CAD build for the part. Positions are in the model's coordinates, mm. A direction names the side the tool comes from. Give positions to 0.01 mm unless a question says otherwise; leave off trailing zeros. Write each loop counter-clockwise with the first axis right and the second up, starting at its lowest first coordinate (ties: lowest second). Pieces come first, ordered by that corner, then holes. Notation, with made-up numbers: (59, 36.25) - (95, 36.25) arc R9 ccw to (95, 49.25) - close; hole circle Ø9 at (4.25, 75). An arc over 180 degrees is marked (long way). Answer as a JSON object with one key per item and string values.
from build123d import *

# Parameters (mm, degrees)
F0_W      = 25
F0_H      = 25
F0_R      = 10.25
F0_R_2    = 9.25
F0_R_3    = 8
F1_DEPTH  = 1
F2_W      = 25
F2_H      = 25
F2_R      = 9.25
F3_DEPTH  = 3
F4_W      = 25
F4_H      = 25
F4_R      = 10.25
F5_DEPTH  = 10
F6_W      = 13
F6_H      = 3
F7_DEPTH  = 10
F8_W      = 7.5
F8_H      = 10
F9_DEPTH  = 3.5
F11_DEPTH = 10
F12_DEPTH = 10


with BuildPart() as f1:
    # F0 (on Front) → F1 (new body)
    with BuildSketch(Plane.XZ):
        with Locations((12.5, 12.5)):
            Rectangle(F0_W, F0_H)
        with Locations((12.5, 12.5)):
            Circle(F0_R, mode=Mode.SUBTRACT)
        with Locations((12.5, 12.5)):
            Circle(F0_R)
        with Locations((12.5, 12.5)):
            Circle(F0_R_2, mode=Mode.SUBTRACT)
        with Locations((12.5, 12.5)):
            Circle(F0_R_2)
        with Locations((12.5, 12.5)):
            Circle(F0_R_3, mode=Mode.SUBTRACT)
    extrude(amount=F1_DEPTH)

    # F2 (on face) → F3 (join)
    with BuildSketch(Plane.XZ.offset(1)):
        with Locations((12.5, 12.5)):
            Rectangle(F2_W, F2_H)
        with Locations((12.5, 12.5)):
            Circle(F2_R, mode=Mode.SUBTRACT)
    extrude(amount=F3_DEPTH)

    # F4 (on face) → F5 (join)
    with BuildSketch(Plane.XZ.offset(4)):
        with Locations((12.5, 12.5)):
            Rectangle(F4_W, F4_H)
        with Locations((12.5, 12.5)):
            Circle(F4_R, mode=Mode.SUBTRACT)
    extrude(amount=F5_DEPTH)

    # F6 (on face) → F7 (join)
    with BuildSketch(Plane.XY.offset(25)):
        with Locations((12.5, -12.5)):
            Rectangle(F6_W, F6_H)
    extrude(amount=F7_DEPTH)

    # F8 (on face) → F9 (join)
    with BuildSketch(Plane.XZ.offset(14)):
        with Locations((12.25, 30)):
            Rectangle(F8_W, F8_H)
    extrude(amount=F9_DEPTH)

    # F10 (on face) → F11 (cut)
    with BuildSketch(Plane.XY.offset(35)):
        Polygon((8.5, -14), (8.5, -17.5), (9.5, -14), align=None)
    extrude(amount=-F11_DEPTH, mode=Mode.SUBTRACT)

    # F10 (on face) → F12 (cut)
    with BuildSketch(Plane.XY.offset(35)):
        Polygon((15, -14), (16, -17.5), (16, -14), align=None)
    extrude(amount=-F12_DEPTH, mode=Mode.SUBTRACT)


solid = f1.part
Item 1: Flat gauge pins, fed straight in: P1, Ø3.5, axis at y = -12, z = 28.5, coming from the +X side; P2, Ø3, axis at x = 14.5, z = 32.5, coming from the +Y side; P3, Ø10, axis at y = -4, z = 18.5, coming from the -X side; P4, Ø1, axis at x = 12.5, y = -15, coming from the -Z side. Where does each tip first touch, or does it go through?
Entries:
{"P1": "x = 19", "P2": "y = -11", "P3": "x = 0", "P4": "z = 25"}
Item 2: Which spindle directions (+Z, -Z, +X, -X, +Y, -Y) get a long thin tool onto all of the face, cutting with end or side? Do faces 5 (the flat face through (15.493, -15.726, 30.07)), 6 (the flat face through (12, -11, 30)), 7 (the flat face through (12, -16, 25)), 8 (the flat face through (11, -4, 22)). Say none if no direction does.
Entries:
{"face 5": "+Z, -Z, +X", "face 6": "+Z, +X, -X, +Y", "face 7": "-Z, +X, -X, -Y", "face 8": "-Y"}
Item 3: Mould opens along Z. For faces 1 (the flat face through (8.993, -15.774, 30.07)), 2 (the flat face through (12, -13, 35)), 3 (the cylindrical face through (10.77, -0.49, 4.69)), 4 (the cylindrical face through (16.768, -2.479, 4.294)) say: +Z half, -Z half, draft (parallel to the pull), parting line (faces both ways), or undercut.
Entries:
{"face 1": "draft", "face 2": "+Z half", "face 3": "undercut", "face 4": "undercut"}
Item 4: Probe line 1 (Z direction, x = 12.5, y = -2.1); line 2 (Z direction, x = 12.5, y = -0.8); line 3 (Y direction, x = 10.5, z = 26). List the from-to ranges inside material, lowest first. Write a range as from..to.
Entries:
{"line 1": "0..3.25, 21.75..25", "line 2": "0..4.5, 20.5..25", "line 3": "-17.5..-11"}
Item 5: Cut at D-D (z = 19). Give the cut face in (x, y), and give its area (3 significant figures).
Entries:
{"outline": "(0, -14) - (4.57, -14) - (4.57, -4) - (5.92, -4) - (5.92, -1) - (7.84, -1) - (7.84, 0) - (0, 0) - close; (17.16, -1) - (19.08, -1) - (19.08, -4) - (20.43, -4) - (20.43, -14) - (25, -14) - (25, 0) - (17.16, 0) - close", "area": "143 mm2"}
Item 6: Cut at B-B (z = 12.5). Give the cut face in (x, y), and give its area (3 significant figures).
Entries:
{"outline": "(0, -14) - (2.25, -14) - (2.25, -4) - (3.25, -4) - (3.25, -1) - (4.5, -1) - (4.5, 0) - (0, 0) - close; (20.5, -1) - (21.75, -1) - (21.75, -4) - (22.75, -4) - (22.75, -14) - (25, -14) - (25, 0) - (20.5, 0) - close", "area": "73.5 mm2"}
Item 7: Cut at C-C (y = -9). Give the cut face in (x, z), and give its area (3 significant figures).
Entries:
{"outline": "(0, 0) - (25, 0) - (25, 25) - (0, 25) - close; hole circle Ø20.5 at (12.5, 12.5)", "area": "295 mm2"}
Item 8: Cut at A-A (x = 12.5). Give the cut face in (y, z), and give its area (4 significant figures).
Entries:
{"outline": "(-17.5, 25) - (-14, 25) - (-14, 22.75) - (-4, 22.75) - (-4, 21.75) - (-1, 21.75) - (-1, 20.5) - (0, 20.5) - (0, 25) - (-11, 25) - (-11, 35) - (-17.5, 35) - close; (-14, 0) - (0, 0) - (0, 4.5) - (-1, 4.5) - (-1, 3.25) - (-4, 3.25) - (-4, 2.25) - (-14, 2.25) - close", "area": "138.5 mm2"}
